```python
from build123d import *

# Parameters (mm, degrees)
SKETCH1_R           = 10
SKETCH1_W           = 20
SKETCH1_H           = 20
BOSS_EXTRUDE1_DEPTH = 25
SKETCH2_R           = 15
SKETCH2_W           = 30
SKETCH2_H           = 30
CUT_EXTRUDE1_DEPTH  = 22
SKETCH3_W           = 20.575
SKETCH3_H           = 3
SKETCH3_W_2         = 3
SKETCH3_H_2         = 20.575
SKETCH3_H_3         = 180
BOSS_EXTRUDE3_DEPTH = 22
BOSS_EXTRUDE4_DEPTH = 22
SKETCH7_W           = 30
SKETCH7_H           = 30
SKETCH7_W_2         = 20
SKETCH7_H_2         = 20
BOSS_EXTRUDE5_DEPTH = 5


with BuildPart() as part:
    # Sketch1 → Boss-Extrude1 (new body)
    with BuildSketch(Plane.XY):
        with BuildLine():
            Line((-35.525235512, -1.881028125), (-24.96502847, -201.321875))
            ThreePointArc((-24.96502847, -201.321875), (0, -225), (24.96502847, -201.321875))
            Line((24.96502847, -201.321875), (35.525235512, -1.881028125))
            ThreePointArc((35.525235512, -1.881028125), (0, 35.575), (-35.525235512, -1.881028125))
        make_face()
        with Locations((0, -200)):
            Circle(SKETCH1_R, mode=Mode.SUBTRACT)
        Rectangle(SKETCH1_W, SKETCH1_H, mode=Mode.SUBTRACT)
    extrude(amount=BOSS_EXTRUDE1_DEPTH)

    # Sketch2 → Cut-Extrude1 (cut)
    with BuildSketch(Plane.XY.offset(25)):
        with BuildLine():
            Line((-30.532229818, -1.616653125), (-19.972022776, -201.0575))
            ThreePointArc((-19.972022776, -201.0575), (0, -220), (19.972022776, -201.0575))
            Line((19.972022776, -201.0575), (30.532229818, -1.616653125))
            ThreePointArc((30.532229818, -1.616653125), (0, 30.575), (-30.532229818, -1.616653125))
        make_face()
        with Locations((0, -200)):
            Circle(SKETCH2_R, mode=Mode.SUBTRACT)
        Rectangle(SKETCH2_W, SKETCH2_H, mode=Mode.SUBTRACT)
    extrude(amount=-CUT_EXTRUDE1_DEPTH, mode=Mode.SUBTRACT)

    # Sketch3 → Boss-Extrude3 (add)
    with BuildSketch(Plane.XY.offset(25)):
        Polygon((-8.939339828, 11.060660172), (-20.559129663, 22.680450007), (-22.680450007, 20.559129663), (-11.060660172, 8.939339828), align=None)
        with Locations((-20.2875, 0)):
            Rectangle(SKETCH3_W, SKETCH3_H)
        with Locations((0, 20.2875)):
            Rectangle(SKETCH3_W_2, SKETCH3_H_2)
        with Locations((20.2875, 0)):
            Rectangle(SKETCH3_W, SKETCH3_H)
        with Locations((0, -100)):
            Rectangle(SKETCH3_W_2, SKETCH3_H_3)
        Polygon((11.060660172, 8.939339828), (22.680450007, 20.559129663), (20.559129663, 22.680450007), (8.939339828, 11.060660172), align=None)
        Polygon((8.939339828, -11.060660172), (28.971494515, -31.092814858), (31.092814858, -28.971494515), (11.060660172, -8.939339828), align=None)
        Polygon((-11.060660172, -8.939339828), (-31.092814858, -28.971494515), (-28.971494515, -31.092814858), (-8.939339828, -11.060660172), align=None)
    extrude(amount=-BOSS_EXTRUDE3_DEPTH)

    # Sketch6 → Boss-Extrude4 (add)
    with BuildSketch(Plane.XY.offset(25)):
        with BuildLine():
            Line((26.124834301, -51.724054412), (1.5, -98.387483985))
            Line((1.5, -98.387483985), (1.5, -105.460941502))
            Line((1.5, -105.460941502), (20.904572897, -151.463673485))
            Line((20.904572897, -151.463673485), (1.5, -182.26134041))
            Line((1.5, -182.26134041), (1.5, -185.075188443))
            ThreePointArc((1.5, -185.075188443), (2.310598263, -185.179030542), (3.11433813, -185.326864752))
            Line((3.11433813, -185.326864752), (22.428014316, -154.673463132))
            Line((22.428014316, -154.673463132), (22.772239511, -148.172400784))
            Line((22.772239511, -148.172400784), (3.158221033, -101.673132803))
            Line((3.158221033, -101.673132803), (27.696425353, -55.173864823))
            Line((27.696425353, -55.173864823), (28.012106126, -49.211894519))
            Line((28.012106126, -49.211894519), (3.349130043, -15))
            Line((3.349130043, -15), (1.5, -15))
            Line((1.5, -15), (1.5, -17.565069267))
            Line((1.5, -17.565069267), (26.124834301, -51.724054412))
        make_face()
        with BuildLine():
            Line((-1.5, -15), (-3.349130043, -15))
            Line((-3.349130043, -15), (-28.012106126, -49.211894519))
            Line((-28.012106126, -49.211894519), (-27.696425353, -55.173864823))
            Line((-27.696425353, -55.173864823), (-3.158221033, -101.673132803))
            Line((-3.158221033, -101.673132803), (-22.772239511, -148.172400784))
            Line((-22.772239511, -148.172400784), (-22.428014316, -154.673463132))
            Line((-22.428014316, -154.673463132), (-3.11433813, -185.326864752))
            ThreePointArc((-3.11433813, -185.326864752), (-2.310598263, -185.179030542), (-1.5, -185.075188443))
            Line((-1.5, -185.075188443), (-1.5, -182.26134041))
            Line((-1.5, -182.26134041), (-20.904572897, -151.463673485))
            Line((-20.904572897, -151.463673485), (-1.5, -105.460941502))
            Line((-1.5, -105.460941502), (-1.5, -98.387483985))
            Line((-1.5, -98.387483985), (-26.124834301, -51.724054412))
            Line((-26.124834301, -51.724054412), (-1.5, -17.565069267))
            Line((-1.5, -17.565069267), (-1.5, -15))
        make_face()
    extrude(amount=-BOSS_EXTRUDE4_DEPTH)

    # Sketch7 → Boss-Extrude5 (add)
    with BuildSketch(Plane.XY.offset(25)):
        Rectangle(SKETCH7_W, SKETCH7_H)
        Rectangle(SKETCH7_W_2, SKETCH7_H_2, mode=Mode.SUBTRACT)
    extrude(amount=BOSS_EXTRUDE5_DEPTH)


solid = part.part
```
The model under review builds one solid part; all positions refer to its coordinate system, in mm. A direction names the side the tool comes from. Coordinates: 2 decimals unless noted, no trailing zeros. Order: outer loops, then holes, each group sorted by start corner. A loop starts at its lowest first (then second) coordinate and runs counter-clockwise, first axis right, second up. Notation, with made-up numbers: (-9, 20.5) -> (4, 20.5) arc R7 cw to (4, 29.5) -> close; hole circle Ø8 at (-17.75, 16). An arc over 180 degrees is marked (long way). Answer in a Markdown table with one row per item. Add a question column.
Item 1: We need section B-B on z = 21. Give the number of separate pieces and of enclosed holes in the cut face, plus the area to 3 significant figures.
Item 2: To check wall thickness, follow probe 1 along Y at (x, z) = (-1, 20.5); probe 2 along Y at (x, z) = (0.5, 2) (1 decimal); probe 3 along X at (y, z) = (-91, 24.75). State the ranges of each line that lie inside material, in increasing order.
Item 3: Clearance check with flat-ended pins moving along their axes: pin 1 (1.5 mm diameter, centred on y = -6, z = 8.5, fed in from +X); pin 2 (9.5 mm diameter, centred on x = -15.5, y = -155, fed in from +Z); pin 3 (7.5 mm diameter, centred on x = 11, y = -54, fed in from +Z); pin 4 (12 mm diameter, centred on x = 4.5, z = 25.5, fed in from -Y). State where each tip first meets the part, or that it passes through.
Item 4: Machinability: for faces 1 (the flat face through (15.853, -32.345, 14.154)), 2 (the flat face through (10, 0, 15)), which of the approach directions +Z, -Z, +X, -X, +Y, -Y give a long, thin tool a straight path to every point of the face, cutting with its end or side? Answer none if there is none.
Item 5: We need section A-A on y = -68.5. Write out the cut boundary in (x, z), plus the area to 3 significant figures.
Item 6: We need section C-C on y = 18. Write out the cut boundary in (x, z).
Item 7: Mouldability with a two-part tool opening along X and no side actions: class faces 3 (the flat face through (-25.27, -101.02, 14.15)), 4 (the flat face through (1.5, -59, 14)), 5 (the cylindrical face through (-0.531, -224.994, 12.325)), 6 (the flat face through (-10.2, 0.2, 30)) as +X half, -X half, draft (parallel to the pull), parting line (faces both ways), or undercut.
Final values:
| question | item | result |
|---|---|---|
| 1 | separate pieces | 1 |
| 1 | enclosed holes | 17 |
| 1 | area | 5,730 mm2 |
| 2 | probe 1 | y = -224.98 to -219.97, -214.97 to -209.95, -190.05 to -10, 10 to 35.56 |
| 2 | probe 2 | y = -225 to -210, -190 to -10, 10 to 35.6 |
| 2 | probe 3 | x = -30.81 to -25.8, -8.79 to -5.4, -1.5 to 1.5, 5.4 to 8.79, 25.8 to 30.81 |
| 3 | pin 1 | stops at x = 35.35 |
| 3 | pin 2 | stops at z = 25 |
| 3 | pin 3 | stops at z = 3 |
| 3 | pin 4 | stops at y = -225 |
| 4 | face 1 | +Z |
| 4 | face 2 | +Z, -Z |
| 5 | outline | (-32, 0) -> (32, 0) -> (32, 25) -> (26.99, 25) -> (26.99, 3) -> (20.66, 3) -> (20.66, 25) -> (17.27, 25) -> (17.27, 3) -> (1.5, 3) -> (1.5, 25) -> (-1.5, 25) -> (-1.5, 3) -> (-17.27, 3) -> (-17.27, 25) -> (-20.66, 25) -> (-20.66, 3) -> (-26.99, 3) -> (-26.99, 25) -> (-32, 25) -> close |
| 5 | area | 628 mm2 |
| 6 | outline | (-30.69, 0) -> (30.69, 0) -> (30.69, 25) -> (24.71, 25) -> (24.71, 3) -> (20.12, 3) -> (20.12, 25) -> (15.88, 25) -> (15.88, 3) -> (1.5, 3) -> (1.5, 25) -> (-1.5, 25) -> (-1.5, 3) -> (-15.88, 3) -> (-15.88, 25) -> (-20.12, 25) -> (-20.12, 3) -> (-24.71, 3) -> (-24.71, 25) -> (-30.69, 25) -> close |
| 7 | face 3 | undercut |
| 7 | face 4 | undercut |
| 7 | face 5 | parting line |
| 7 | face 6 | draft |
